Autodesk Inventor part; units mm, degrees
ref_plane "YZ Plane" through (0, 0, 0) normal (1, 0, 0) x (0, 1, 0)
ref_plane "XZ Plane" through (0, 0, 0) normal (0, 1, 0) x (-1, 0, 0)
ref_plane "XY Plane" through (0, 0, 0) normal (0, 0, 1) x (1, 0, 0)
sketch "Sketch1" plane through (0, 0, 0) normal (0, 1, 0) x (-1, 0, 0)
  line L0 (0, 0) -> (-254, 0)
  line L1 (-254, 0) -> (-254, -254)
  line L2 (-254, -254) -> (0, -254)
  line L3 (0, -254) -> (0, 0)
  line L4 (0, -15.875) -> (-10.287, -15.875)
  line L5 (-10.287, -15.875) -> (-10.287, 0)
  line L6 (-243.713, 0) -> (-243.713, -15.875)
  line L7 (-243.713, -15.875) -> (-254, -15.875)
  line L8 (-243.713, -254) -> (-243.713, -238.125)
  line L9 (-243.713, -238.125) -> (-254, -238.125)
  line L10 (-10.287, -254) -> (-10.287, -238.125)
  line L11 (-10.287, -238.125) -> (0, -238.125)
  dimension "d0" = 254
  dimension "d1" = 254
  dimension "d13" = 10.287
  dimension "d14" = 10.287
  dimension "d15" = 15.875
  dimension "d16" = 15.875
extrude "Extrusion1" add sketch "Sketch1" along normal blind 12.7 contours L5 L4 L3 L11 L10 L2 L8 L9 L1 L7 L6 L0
sketch "Sketch2" plane through (0, 12.7, 0) normal (0, 1, 0) x (1, 0, 0)
  line L0 (28.575, 31.75) -> (211.9884, 31.75)
  line L1 (211.9884, 31.75) -> (211.9884, 222.25)
  line L2 (211.9884, 222.25) -> (28.575, 222.25)
  line L3 (28.575, 222.25) -> (28.575, 31.75)
  line L4 (0, 15.875) -> (10.287, 15.875)
  line L5 (10.287, 15.875) -> (10.287, 0)
  line L6 (10.287, 0) -> (243.713, 0)
  line L7 (243.713, 0) -> (243.713, 15.875)
  line L8 (243.713, 15.875) -> (254, 15.875)
  line L9 (254, 15.875) -> (254, 238.125)
  line L10 (254, 238.125) -> (243.713, 238.125)
  line L11 (243.713, 238.125) -> (243.713, 254)
  line L12 (243.713, 254) -> (10.287, 254)
  line L13 (10.287, 254) -> (10.287, 238.125)
  line L14 (10.287, 238.125) -> (0, 238.125)
  line L15 (0, 238.125) -> (0, 15.875)
  point P0 (0, 0)
  point P1 (127, 0)
  point P2 (28.575, 127)
  point P3 (0, 127)
  dimension "d9" = 190.5
  dimension "d29" = 28.575
  dimension "d30" = 42.0116
extrude "Extrusion2" cut sketch "Sketch2" against normal through all contours L3 L2 L1 L0
sketch "Sketch3" plane through (0, 12.7, 0) normal (0, 1, 0) x (1, 0, 0)
  circle A0 centre (50.8, 9.525) radius 7.5
  circle A1 centre (50.8, 244.475) radius 7.5
  circle A2 centre (203.2, 244.475) radius 4
  circle A3 centre (203.2, 244.475) radius 7.5
  circle A4 centre (203.2, 9.525) radius 7.5
  point P0 (0, 0)
hole "Hole1" at (50.8, 12.7, -9.525) at (50.8, 12.7, -244.475) at (203.2, 12.7, -9.525) at (203.2, 12.7, -244.475) direction (0, -1, 0) diameter 15 end through all
chamfer "Chamfer1" distance 3.175 angle 45 1 edges at (0, 6.35, -238.125)
equation "\"d14\" = d13"
properties part number "Carriage Sheet"
Part model, mm, in its own coordinate system. A direction names the side the tool comes from. Round coordinates to 2 decimals unless told otherwise and drop trailing zeros. Loops run counter-clockwise (first coordinate to the right, second up) from the corner with the lowest first, then second, coordinate; pieces in that order, holes last.
1. Flat gauge pins, fed straight in: pin 1 (6.5 mm diameter, centred on y = 9, z = -248, fed in from +X); pin 2 (3 mm diameter, centred on x = 250.5, y = 9, fed in from +Z) (3 decimals); pin 3 (2 mm diameter, centred on x = 7, y = 9.5, fed in from -Z) (3 decimals). Where does each tip first touch, or does it go through?
Solutions:
pin 1: stops at x = 243.71
pin 2: stops at z = -15.875
pin 3: stops at z = -238.125
2. Drill centre lines: line 1 along X through (y, z) = (8.5, -123) (3 decimals); line 2 along Z through (x, y) = (70, 7.25); line 3 along Z through (x, y) = (49, 12.25). Where is each one in solid material? Low to high.
Solutions:
line 1: x = 0 to 28.575, 211.988 to 254
line 2: z = -254 to -222.25, -31.75 to 0
line 3: z = -254 to -251.76, -237.19 to -222.25, -31.75 to -16.81, -2.24 to 0
3. Slice it at C-C (x = 150.5). Give the cut face in (y, z).
Solutions:
outline: (0, -254) - (12.7, -254) - (12.7, -222.25) - (0, -222.25) - close; (0, -31.75) - (12.7, -31.75) - (12.7, 0) - (0, 0) - close
4. 3-axis set-ups, long thin cutter, end or side, ignore diameter. For faces 5 (the face through (5, 6, -15.875)), 6 (the face through (10.287, 6, -246)), 7 (the face through (211.988, 6, -126)), 8 (the face through (243.713, 6, -8)), 9 (the face through (243.713, 6, -246)): which of +Z, -Z, +X, -X, +Y, -Y reach the whole face in a straight line?
Solutions:
face 5: +Z, -X, +Y, -Y
face 6: -Z, -X, +Y, -Y
face 7: +Y, -Y
face 8: +Z, +X, +Y, -Y
face 9: -Z, +X, +Y, -Y
5. Slice it at A-A (y = 6). Give the cut face in (x, z) (3 decimals).
Solutions:
outline: (0, -234.95) - (3.175, -238.125) - (10.287, -238.125) - (10.287, -254) - (243.713, -254) - (243.713, -238.125) - (254, -238.125) - (254, -15.875) - (243.713, -15.875) - (243.713, 0) - (10.287, 0) - (10.287, -15.875) - (0, -15.875) - close; hole (28.575, -222.25) - (211.988, -222.25) - (211.988, -31.75) - (28.575, -31.75) - close; hole circle Ø15 at (50.8, -244.475); hole circle Ø15 at (50.8, -9.525); hole circle Ø15 at (203.2, -244.475); hole circle Ø15 at (203.2, -9.525)
6. Slice it at B-B (z = -45). Give the cut face in (x, y) (3 decimals), and give its area (3 significant figures).
Solutions:
outline: (0, 0) - (28.575, 0) - (28.575, 12.7) - (0, 12.7) - close; (211.988, 0) - (254, 0) - (254, 12.7) - (211.988, 12.7) - close
area: 896 mm2
7. Two-plate mould, pull along X, no slides. Class faces 1 (the face through (122, 6, -222.25)), 2 (the face through (0, 6, -127)), 3 (the face through (206.073, 6.261, -237.547)), 4 (the face through (213, 12.7, -125)): pulls with the +X half, pulls with the -X half, needs draft (parallel to the pull), parting line crosses it, or undercut.
Solutions:
face 1: undercut
face 2: pulls with the -X half
face 3: undercut
face 4: needs draft
8. Slice it at D-D (x = 203.2). Give the cut face in (y, z) (3 decimals).
Solutions:
outline: (0, -254) - (12.7, -254) - (12.7, -251.975) - (0, -251.975) - close; (0, -236.975) - (12.7, -236.975) - (12.7, -222.25) - (0, -222.25) - close; (0, -31.75) - (12.7, -31.75) - (12.7, -17.025) - (0, -17.025) - close; (0, -2.025) - (12.7, -2.025) - (12.7, 0) - (0, 0) - close
